from build123d import *

# Parameters (mm, degrees)
F0_W      = 70
F0_H      = 48
F1_DEPTH  = 25
F2_R      = 30
F3_DEPTH  = 9
F4_R      = 28
F5_DEPTH  = 25
F6_R      = 4.25
F7_DEPTH  = 25
F9_DEPTH  = 25
F11_DEPTH = 25
F13_DEPTH = 75


with BuildPart() as f1:
    # F0 (on Right) → F1 (new body)
    with BuildSketch(Plane.YZ):
        Rectangle(F0_W, F0_H)
    extrude(amount=F1_DEPTH)

    # F2 (on face) → F3 (cut)
    with BuildSketch(Plane.YZ.offset(25)):
        with Locations((0, 24)):
            Circle(F2_R)
    extrude(amount=-F3_DEPTH, mode=Mode.SUBTRACT)

    # F4 (on face) → F5 (cut)
    with BuildSketch(Plane.YZ.offset(16)):
        with Locations((0, 24)):
            Circle(F4_R)
    extrude(amount=-F5_DEPTH, mode=Mode.SUBTRACT)

    # F6 (on face) → F7 (cut)
    with BuildSketch(Plane(origin=(0, 0, -24), x_dir=(1, 0, 0), z_dir=(0, 0, -1))):
        with Locations((8, 0)):
            Circle(F6_R)
    extrude(amount=-F7_DEPTH, mode=Mode.SUBTRACT)

    # F8 (on face) → F9 (cut)
    with BuildSketch(Plane.XY.offset(24)):
        Polygon((8, -28), (8, -32.5), (20, -32.5), (20, -27.5), (20, -10), (8, -10), align=None)
    extrude(amount=-F9_DEPTH, mode=Mode.SUBTRACT)

    # F10 (on face) → F11 (cut)
    with BuildSketch(Plane.YZ.offset(25)):
        with BuildLine():
            Line((25, -30.528549), (25, -24))
            ThreePointArc((25, -24), (0, -12.129655), (-25, -24))
            Line((-25, -24), (-25, -30.528549))
            Line((-25, -30.528549), (25, -30.528549))
        make_face()
    extrude(amount=-F11_DEPTH, mode=Mode.SUBTRACT)

    # F12 (on face) → F13 (cut)
    with BuildSketch(Plane.XZ.offset(35)):
        with BuildLine():
            Line((20, -27.683428), (20, -24))
            ThreePointArc((20, -24), (12.5, -19.900788), (5, -24))
            Line((5, -24), (5, -27.683428))
            Line((5, -27.683428), (20, -27.683428))
        make_face()
    extrude(amount=-F13_DEPTH, mode=Mode.SUBTRACT)


solid = f1.part
The model under review builds one solid part; all positions refer to its coordinate system, in mm. A direction names the side the tool comes from. Coordinates: 2 decimals unless noted, no trailing zeros. Write each loop counter-clockwise with the first axis right and the second up, starting at its lowest first coordinate (ties: lowest second). Pieces come first, ordered by that corner, then holes. Notation, with made-up numbers: (-30, 18) -> (12, 18) arc R15 ccw to (12, 25) -> close; hole circle Ø4 at (-0.5, 46). An arc over 180 degrees is marked (long way). Answer in a Markdown table with one row per item.
1. We need section C-C, the plane z = 16.5. State the section outline as (x, y) points, and give its area (3 significant figures).
Answers below:
| item | result |
|---|---|
| outline | (0, -35) -> (25, -35) -> (25, -29.05) -> (20, -29.05) -> (20, -32.5) -> (8, -32.5) -> (8, -26.98) -> (0, -26.98) -> close; (0, 26.98) -> (16, 26.98) -> (16, 29.05) -> (25, 29.05) -> (25, 35) -> (0, 35) -> close |
| area | 306 mm^2 |
2. For faces 5 (the cylindrical face through (20.56, 9.64, -4.41)), 6 (the cylindrical face through (4.868, -2.872, -8.104)), 7 (the flat face through (20, -28, 9)), list the 3-axis set-ups (+Z, -Z, +X, -X, +Y, -Y) from which the entire face can be reached by the end or side of a thin tool; tool diameter is ignored.
Answers below:
| item | result |
|---|---|
| face 5 | +Z, +X |
| face 6 | +Z, -Z |
| face 7 | +Z |
3. Clearance check with flat-ended pins moving along their axes: pin 1 Ø10 at (y, z) = (18, -18) entering from -X; pin 2 Ø3 at (x, y) = (5.5, -20) entering from +Z; pin 3 Ø10 at (x, y) = (8, 0) entering from -Z; pin 4 Ø2 at (y, z) = (-12.5, -16) entering from +X. State where each tip first meets the part, or that it passes through.
Answers below:
| item | result |
|---|---|
| pin 1 | stops at x = 0 |
| pin 2 | stops at z = 6.06 |
| pin 3 | stops at z = -12.52 |
| pin 4 | passes through |
4. Wall thickness on probe 1 along X at (y, z) = (0, -8); probe 2 along Y at (x, z) = (8, -7.75); probe 3 along X at (y, z) = (0, -5.75): over which ranges is each line inside the solid? List them lowest first. Write a range as [from, to].
Answers below:
| item | result |
|---|---|
| probe 1 | x = [0, 3.75], [12.25, 25] |
| probe 2 | y = [-35, -4.25], [4.25, 35] |
| probe 3 | x = [0, 3.75], [12.25, 16] |
5. Draft analysis for pull direction X (two halves, no side actions). For faces 1 (the flat face through (8, -27, 9)), 2 (the flat face through (0, 0, -5)), 3 (the cylindrical face through (12.6, -28.1, -19.9)), 4 (the flat face through (12, 31, 24)), state which applies: +X half, -X half, draft (parallel to the pull), parting line (faces both ways), or undercut.
Answers below:
| item | result |
|---|---|
| face 1 | undercut |
| face 2 | -X half |
| face 3 | undercut |
| face 4 | draft |
6. We need section D-D, the plane x = 22.25. State the section outline as (y, z) points.
Answers below:
| item | result |
|---|---|
| outline | (-35, -24) -> (-25, -24) arc R32.26 cw to (25, -24) -> (35, -24) -> (35, 24) -> (30, 24) arc R30 cw to (-30, 24) -> (-35, 24) -> close |
7. We need section B-B, the plane y = 0. State the section outline as (x, z) points.
Answers below:
| item | result |
|---|---|
| outline | (0, -12.13) -> (3.75, -12.13) -> (3.75, -4) -> (0, -4) -> close; (12.25, -12.13) -> (25, -12.13) -> (25, -6) -> (16, -6) -> (16, -4) -> (12.25, -4) -> close |
8. We need section A-A, the plane z = -10.5. State the section outline as (x, y) points.
Answers below:
| item | result |
|---|---|
| outline | (0, -35) -> (25, -35) -> (25, 35) -> (0, 35) -> close; hole circle Ø8.5 at (8, 0) |
